```python
from build123d import *

# Parameters (mm, degrees)
BOSS_EXTRUDE1_DEPTH = 4.7625
BOSS_EXTRUDE2_DEPTH = 10.16
BOSS_EXTRUDE3_START = 6.35
BOSS_EXTRUDE3_DEPTH = 6.35
REVOLVE1_ANGLE      = 4


with BuildPart() as part:
    # Sketch1 → Boss-Extrude1 (new body)
    with BuildSketch(Plane(origin=(0, 0, 0), x_dir=(1, 0, 0), z_dir=(0, 1, 0))):
        with BuildLine():
            Line((-201.832488243, -290.825801155), (-206.177018076, -297.085949758))
            ThreePointArc((-206.177018076, -297.085949758), (-195.683270483, -304.100447187), (-184.951112968, -310.744445064))
            Line((-184.951112968, -310.744445064), (-181.053852083, -304.196486787))
            ThreePointArc((-181.053852083, -304.196486787), (-191.559863256, -297.692490193), (-201.832488243, -290.825801155))
        make_face()
    extrude(amount=BOSS_EXTRUDE1_DEPTH)

    # Sketch2 → Boss-Extrude2 (add)
    with BuildSketch(Plane(origin=(0, 4.7625, 0), x_dir=(1, 0, 0), z_dir=(0, 1, 0))):
        with BuildLine():
            Line((-206.177018076, -297.085949758), (-181.558015689, -261.611774341))
            Line((-181.558015689, -261.611774341), (-162.86663462, -273.639348162))
            Line((-162.86663462, -273.639348162), (-184.951112968, -310.744445064))
            ThreePointArc((-184.951112968, -310.744445064), (-195.683270483, -304.100447187), (-206.177018076, -297.085949758))
        make_face()
    extrude(amount=BOSS_EXTRUDE2_DEPTH)

    # Sketch3 → Boss-Extrude3 (add)
    with BuildSketch(Plane.XZ.offset(BOSS_EXTRUDE3_START)):
        with BuildLine():
            ThreePointArc((-184.951112968, 310.744445064), (-195.683270483, 304.100447187), (-206.177018076, 297.085949758))
            Line((-206.177018076, 297.085949758), (-201.832488243, 290.825801155))
            ThreePointArc((-201.832488243, 290.825801155), (-191.559863256, 297.692490193), (-181.053852083, 304.196486787))
            Line((-181.053852083, 304.196486787), (-184.951112968, 310.744445064))
        make_face()
        with BuildLine():
            Line((-162.86663462, 273.639348162), (-181.053852083, 304.196486787))
            ThreePointArc((-181.053852083, 304.196486787), (-191.559863256, 297.692490193), (-201.832488243, 290.825801155))
            Line((-201.832488243, 290.825801155), (-181.558015689, 261.611774341))
            Line((-181.558015689, 261.611774341), (-162.86663462, 273.639348162))
        make_face()
    extrude(amount=-BOSS_EXTRUDE3_DEPTH)

    # Sketch4 → Revolve1 (revolve)
    with BuildSketch(Plane(origin=(0, 0, 0), x_dir=(-0.5701482720363652, 0, 0.8215418114094662), z_dir=(-0.8215418114094664, 0, -0.5701482720363652))):
        Polygon((318.439999898, 1), (353.999999898, 0), (318.439999898, 0), align=None)
    revolve(axis=Axis((0, 0, 0), (0, 1, 0)), revolution_arc=REVOLVE1_ANGLE)


solid = part.part
```
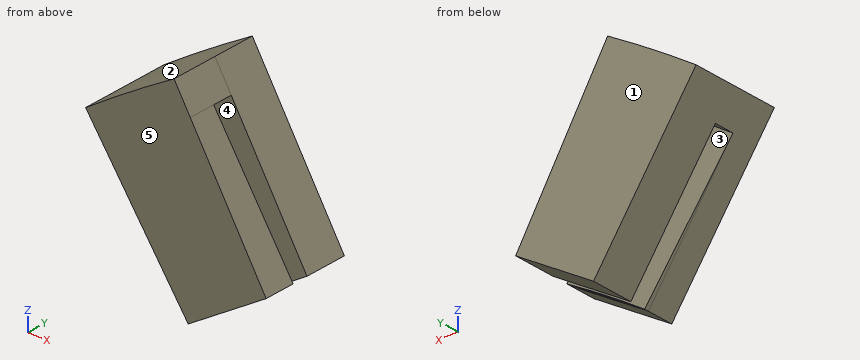
Part model, mm, in its own coordinate system. Face numbers are marked on the shaded views. A direction names the side the tool comes from. Round coordinates to 2 decimals unless told otherwise and drop trailing zeros. Order: outer loops, then holes, each group sorted by start corner. A loop starts at its lowest first (then second) coordinate and runs counter-clockwise, first axis right, second up. Notation, with made-up numbers: M -20,-5.75 L 14,-5.75 A15 cw 14,-1.75 Z; hole C 23.5,86.25 d7. An arc over 180 degrees is marked long. Answer in a Markdown table with one row per item. Add a question column.
Q1. 3-axis set-ups, long thin cutter, end or side, ignore diameter. For the marked faces 4 and 5: which of +Z, -Z, +X, -X, +Y, -Y reach the whole face in a straight line?
Q2. Mould opens along Z. For the marked faces 1, 2 and 3 say: +Z half, -Z half, draft (parallel to the pull), parting line (faces both ways), or undercut.
Q3. Wall check: L1, parallel to Y at x = -181, z = 304; L2, parallel to Y at x = -193, z = 290; L3, parallel to Z at x = -197, y = 5.5. Give the ranges that are in metal, low to high. Write a range as from..to.
Q4. Cut at B-B on z = 306.5. Give the cut face in (x, y), and give its area (3 significant figures).
Q5. Pin check, flat tips, straight feed: pin 1 (5 mm diameter, centred on y = 7.5, z = 270, fed in from +X); pin 2 (6 mm diameter, centred on x = -167.5, y = 0, fed in from -Z); pin 3 (12 mm diameter, centred on y = -2, z = 279, fed in from -X). Stop position of each tip, or through.
Q6. Cut at A-A on y = 2.75. Give the cut face in (x, z).
Established:
| question | item | result |
|---|---|---|
| 1 | face 4 | -Z, +X |
| 1 | face 5 | +Z, -Z, +X, -X, -Y |
| 2 | face 1 | draft |
| 2 | face 2 | +Z half |
| 2 | face 3 | undercut |
| 3 | L1 | y = -6.35..0.01, 4.76..14.92 |
| 3 | L2 | y = -6.35..0.16, 4.76..14.92 |
| 3 | L3 | z = 283.86..303.25 |
| 4 | outline | M -191.9,-6.35 L -182.42,-6.35 L -182.42,14.92 L -191.9,14.92 Z |
| 4 | area | 202 mm2 |
| 5 | pin 1 | stops at x = -164.64 |
| 5 | pin 2 | stops at z = 268.73 |
| 5 | pin 3 | stops at x = -197.79 |
| 6 | outline | M -206.18,297.09 L -201.83,290.83 A354 cw -181.05,304.2 L -184.95,310.74 A361.62 ccw Z |
